Here's how the part is built. I have some questions about the finished solid (model axes, mm). A direction names the side the tool comes from. Coordinates: 2 decimals unless noted, no trailing zeros. Write each loop counter-clockwise with the first axis right and the second up, starting at its lowest first coordinate (ties: lowest second). Pieces come first, ordered by that corner, then holes. Notation, with made-up numbers: (2, 38.5) -> (37, 38.5) arc R21 ccw to (37, 77.5) -> close; hole circle Ø10 at (-25.75, 13). An arc over 180 degrees is marked (long way). Answer in a Markdown table with one row per item. Add a question column.
from build123d import *

# Parameters (mm, degrees)
SKETCH1_W                = 50.8
SKETCH1_H                = 34.925
BOSS_EXTRUDE1_DEPTH      = 3.53568
BOSS_EXTRUDE2_START      = -3.53568
BOSS_EXTRUDE2_DEPTH      = 38.1
CUT_EXTRUDE1_DEPTH       = 66.857337528
F_5_16_CLEARANCE_HOLE1_D = 8.2042


with BuildPart() as part:
    # Sketch1 → Boss-Extrude1 (new body)
    with BuildSketch(Plane(origin=(0, 0, 0), x_dir=(1, 0, 0), z_dir=(0, 1, 0))):
        Rectangle(SKETCH1_W, SKETCH1_H)
    extrude(amount=BOSS_EXTRUDE1_DEPTH)

    # Sketch2 → Boss-Extrude2 (add)
    with BuildSketch(Plane(origin=(0, 3.53568, 0), x_dir=(1, 0, 0), z_dir=(0, 1, 0)).offset(BOSS_EXTRUDE2_START)):
        Polygon((21.86432, -17.4625), (25.4, -17.4625), (25.4, 17.4625), (-25.4, 17.4625), (-25.4, -17.4625), (-21.86432, -17.4625), (-21.86432, 13.92682), (21.86432, 13.92682), align=None)
    extrude(amount=BOSS_EXTRUDE2_DEPTH)

    # Sketch3 → Cut-Extrude1 (cut, through all)
    with BuildSketch(Plane(origin=(25.4, 0, 0), x_dir=(0, 0, -1), z_dir=(1, 0, 0))):
        Polygon((-17.4625, 3.53568), (13.92682, 38.1), (-17.4625, 38.1), align=None)
    extrude(amount=-CUT_EXTRUDE1_DEPTH, mode=Mode.SUBTRACT)

    # 5/16 Clearance Hole1 (through all)
    with Locations(Plane(origin=(0, 3.53568, 0), x_dir=(1, 0, 0), z_dir=(0, 1, 0))):
        with Locations((0, 4.40182)):
            Hole(F_5_16_CLEARANCE_HOLE1_D / 2)


solid = part.part
Q1. For faces 1 (the flat face through (-23.607, 20.576, 1.988)), 2 (the flat face through (21.864, 17, -2)), which set-ups out of +Z, -Z, +X, -X, +Y, -Y let a thin tool reach every point of the face, with its end or its side?
Q2. Imagine slicing it at B-B on z = -3.5. Please give me the cut outline in (x, y), plus the area to 3 significant figures.
Q3. Imagine slicing it at D-D on x = -7.5. Please give me the cut outline in (y, z), plus the area to 3 significant figures.
Q4. Imagine slicing it at A-A on x = 0. Please give me the cut outline in (y, z), plus the area to 3 significant figures.
Q5. I need wall thicknesses on line 1 (X direction, y = 27, z = -12.5); line 2 (Z direction, x = 0, y = 1.75); line 3 (Y direction, x = 11, z = 13). Which ranges of each line are inside material? Lowest first, please. Write a range as [from, to].
Q6. Imagine slicing it at C-C on y = 24. Please give me the cut outline in (x, z).
Q7. If we mould it in two halves opening along X, with no side actions, what happens to faces 3 (the flat face through (25.4, 15, -4)), 4 (the flat face through (0, 3.536, 2)), 5 (the flat face through (0, 21, -13.927)), 6 (the flat face through (0, 2, 17.462))? For each: pulls with the +X half, pulls with the -X half, needs draft (parallel to the pull), parting line crosses it, or undercut.
Q8. I'm going to push flat-ended pins straight in: P1, Ø10, axis at x = 2.5, z = 5.5, coming from the -Y side; P2, Ø1, axis at x = -8.5, y = 18.5, coming from the +Z side; P3, Ø1.5, axis at x = 6, z = -3, coming from the +Y side. Where does each tip first touch, or does it pass through?
Result sheet:
| question | item | result |
|---|---|---|
| 1 | face 1 | +Z, +X, -X, +Y |
| 1 | face 2 | +Z, +Y |
| 2 | outline | (-25.4, 0) -> (-4, 0) -> (-4, 3.54) -> (-21.86, 3.54) -> (-21.86, 26.62) -> (-25.4, 26.62) -> close; (4, 0) -> (25.4, 0) -> (25.4, 26.62) -> (21.86, 26.62) -> (21.86, 3.54) -> (4, 3.54) -> close |
| 2 | area | 315 mm^2 |
| 3 | outline | (0, -17.46) -> (38.1, -17.46) -> (38.1, -13.93) -> (3.54, -13.93) -> (3.54, 17.46) -> (0, 17.46) -> close |
| 3 | area | 246 mm^2 |
| 4 | outline | (0, -17.46) -> (38.1, -17.46) -> (38.1, -13.93) -> (3.54, -13.93) -> (3.54, -8.5) -> (0, -8.5) -> close; (0, -0.3) -> (3.54, -0.3) -> (3.54, 17.46) -> (0, 17.46) -> close |
| 4 | area | 217 mm^2 |
| 5 | line 1 | x = [-25.4, -21.86], [21.86, 25.4] |
| 5 | line 2 | z = [-17.46, -8.5], [-0.3, 17.46] |
| 5 | line 3 | y = [0, 3.54] |
| 6 | outline | (-25.4, -17.46) -> (25.4, -17.46) -> (25.4, -1.12) -> (21.86, -1.12) -> (21.86, -13.93) -> (-21.86, -13.93) -> (-21.86, -1.12) -> (-25.4, -1.12) -> close |
| 7 | face 3 | pulls with the +X half |
| 7 | face 4 | undercut |
| 7 | face 5 | undercut |
| 7 | face 6 | needs draft |
| 8 | P1 | stops at y = 0 |
| 8 | P2 | stops at z = -13.93 |
| 8 | P3 | stops at y = 3.54 |
